Input: part model. Units: mm. Frame: model coordinates. A direction names the side the tool comes from. Coordinates: 2 decimals unless noted, no trailing zeros. Order: outer loops, then holes, each group sorted by start corner. A loop starts at its lowest first (then second) coordinate and runs counter-clockwise, first axis right, second up.
from build123d import *

# Parameters (mm, degrees)
F1_DEPTH = 4.064
F3_DEPTH = 15.24
F4_DEPTH = 15.24


with BuildPart() as f1:
    # F0 (on Top) → F1 (new body)
    with BuildSketch(Plane.XY):
        with BuildLine():
            Line((14.976974, 10.16), (-14.976974, 10.16))
            ThreePointArc((-14.976974, 10.16), (-15.219978, 10.111664), (-15.425987, 9.974013))
            Line((-15.425987, 9.974013), (-25.214013, 0.185987))
            ThreePointArc((-25.214013, 0.185987), (-25.351664, -0.020022), (-25.4, -0.263026))
            Line((-25.4, -0.263026), (-25.4, -1.251))
            Line((-25.4, -1.251), (-25.4, -19.685))
            ThreePointArc((-25.4, -19.685), (-25.214013, -20.134013), (-24.765, -20.32))
            Line((-24.765, -20.32), (24.765, -20.32))
            ThreePointArc((24.765, -20.32), (25.214013, -20.134013), (25.4, -19.685))
            Line((25.4, -19.685), (25.4, -0.263026))
            ThreePointArc((25.4, -0.263026), (25.351664, -0.020022), (25.214013, 0.185987))
            Line((25.214013, 0.185987), (15.425987, 9.974013))
            ThreePointArc((15.425987, 9.974013), (15.219978, 10.111664), (14.976974, 10.16))
        make_face()
    extrude(amount=F1_DEPTH)

    # F2 (on face) → F3 (join)
    with BuildSketch(Plane.XY.offset(4.064)):
        with BuildLine():
            Line((-25.4, -0.263026), (-25.4, -19.685))
            ThreePointArc((-25.4, -19.685), (-25.214013, -20.134013), (-24.765, -20.32))
            Line((-24.765, -20.32), (24.765, -20.32))
            ThreePointArc((24.765, -20.32), (25.214013, -20.134013), (25.4, -19.685))
            Line((25.4, -19.685), (25.4, -0.263026))
            Line((25.4, -0.263026), (-25.4, -0.263026))
        make_face()
    extrude(amount=-F3_DEPTH)

    # F2 (on face) → F4 (join)
    with BuildSketch(Plane.XY.offset(4.064)):
        with BuildLine():
            Line((-25.4, -0.263026), (-25.4, -19.685))
            ThreePointArc((-25.4, -19.685), (-25.214013, -20.134013), (-24.765, -20.32))
            Line((-24.765, -20.32), (24.765, -20.32))
            ThreePointArc((24.765, -20.32), (25.214013, -20.134013), (25.4, -19.685))
            Line((25.4, -19.685), (25.4, -0.263026))
            Line((25.4, -0.263026), (-25.4, -0.263026))
        make_face()
    extrude(amount=-F4_DEPTH)


solid = f1.part
Item 1: Cut plane C-C on y = 6.5. Return loops of the section in (x, z).
Response values:
outline: (-18.9, 0) - (18.9, 0) - (18.9, 4.06) - (-18.9, 4.06) - close
Item 2: Ray query, probe 1 along Z at (x, y) = (-22.5, 2.5); probe 2 along Y at (x, z) = (-12, -5.75); probe 3 along Y at (x, z) = (-22, 0.5). Return the intervals inside material, ascending.
Response values:
probe 1: z = 0 to 4.06
probe 2: y = -20.32 to -0.26
probe 3: y = -20.32 to 3.4
Item 3: Cut plane A-A on z = -1.5. Return loops of the section in (x, y) (3 decimals).
Response values:
outline: (-25.4, -19.685) arc R0.635 ccw to (-24.765, -20.32) - (24.765, -20.32) arc R0.635 ccw to (25.4, -19.685) - (25.4, -0.263) - (-25.4, -0.263) - close
Item 4: Access query for faces 1 (the face through (0, -0.263, -6)), 2 (the face through (0, 10.16, 2)). Directions: +Z, -Z, +X, -X, +Y, -Y. A direction counts if a zero-diameter tool reaches every point of the face in a straight line with its end or side. Return the directions, or none.
Response values:
face 1: -Z, +X, -X, +Y
face 2: +Z, -Z, +X, -X, +Y
Item 5: Cut plane B-B on x = 11. Return loops of the section in (y, z), then the cut area to 3 significant figures.
Response values:
outline: (-20.32, -11.18) - (-0.26, -11.18) - (-0.26, 0) - (10.16, 0) - (10.16, 4.06) - (-20.32, 4.06) - close
area: 348 mm2
Item 6: Pin query (flat end, axial travel): pin 1 Ø8.5 at (x, y) = (-5, 4.5) entering from -Z. Return the tip coordinate at first contact, or that it passes through.
Response values:
pin 1: stops at z = 0
